```python
from build123d import *
from OCP.BRepFilletAPI import BRepFilletAPI_MakeChamfer

# Parameters (mm, degrees)
SKETCH1_W          = 20.32
SKETCH1_H          = 40.64
EXTRUDE1_DEPTH     = 29.2
SKETCH2_W          = 20.32
SKETCH2_H          = 40.64
EXTRUDE2_DEPTH     = 2.38125
SKETCH3_W          = 20.32
SKETCH3_H          = 40.64
EXTRUDE3_DEPTH     = 8.2
EXTRUDE6_DEPTH     = 0.635
CHAMFER2_SIZE      = 2.54
CHAMFER2_SIZE2     = 1.466469684
FILLET1_R          = 1.016
FILLET2_R          = 1.524
SKETCH9_W          = 6.35
SKETCH9_H          = 2.54
EXTRUDE8_DEPTH     = 2.38125
SKETCH10_W         = 5.08
SKETCH10_H         = 1.27
CUT_EXTRUDE1_DEPTH = 2.38125
SKETCH_1_R         = 6.5
EXTRUDE_1_DEPTH    = 2
EXTRUDE_1_TAPER    = 9
FILLET_1_R         = 0.5
SKETCH_2_R         = 2.5
EXTRUDE_2_DEPTH    = 4


with BuildPart() as part:
    # Sketch1 → Extrude1 (new body)
    with BuildSketch(Plane(origin=(0, 0, 0), x_dir=(1, 0, 0), z_dir=(0, 1, 0))):
        with Locations((0, -10.16)):
            Rectangle(SKETCH1_W, SKETCH1_H)
    extrude(amount=EXTRUDE1_DEPTH)

    # Sketch2 → Extrude2 (add)
    with BuildSketch(Plane(origin=(0, 29.2, 0), x_dir=(-1, 0, 0), z_dir=(0, 1, 0))):
        with Locations((0, 10.16)):
            Rectangle(SKETCH2_W, SKETCH2_H)
        with BuildLine():
            ThreePointArc((6.731, -15.51418631), (5.08, -11.7094), (3.429, -15.51418631))
            Line((3.429, -15.51418631), (3.429, -16.4846))
            Line((3.429, -16.4846), (-3.429, -16.4846))
            Line((-3.429, -16.4846), (-3.429, -15.51418631))
            ThreePointArc((-3.429, -15.51418631), (-5.08, -11.7094), (-6.731, -15.51418631))
            Line((-6.731, -15.51418631), (-6.731, -16.4846))
            Line((-6.731, -16.4846), (-10.16, -16.4846))
            Line((-10.16, -16.4846), (-10.16, -10.16))
            Line((-10.16, -10.16), (10.16, -10.16))
            Line((10.16, -10.16), (10.16, -16.4846))
            Line((10.16, -16.4846), (6.731, -16.4846))
            Line((6.731, -16.4846), (6.731, -15.51418631))
        make_face()
        with BuildLine():
            ThreePointArc((-6.731, 35.83418631), (-5.08, 32.0294), (-3.429, 35.83418631))
            Line((-3.429, 35.83418631), (-3.429, 36.8046))
            Line((-3.429, 36.8046), (3.429, 36.8046))
            Line((3.429, 36.8046), (3.429, 35.83418631))
            ThreePointArc((3.429, 35.83418631), (5.08, 32.0294), (6.731, 35.83418631))
            Line((6.731, 35.83418631), (6.731, 36.8046))
            Line((6.731, 36.8046), (10.16, 36.8046))
            Line((10.16, 36.8046), (10.16, 30.48))
            Line((10.16, 30.48), (-10.16, 30.48))
            Line((-10.16, 30.48), (-10.16, 36.8046))
            Line((-10.16, 36.8046), (-6.731, 36.8046))
            Line((-6.731, 36.8046), (-6.731, 35.83418631))
        make_face()
    extrude(amount=EXTRUDE2_DEPTH)

    # Sketch3 → Extrude3 (add)
    with BuildSketch(Plane(origin=(0, 31.58125, 0), x_dir=(-1, 0, 0), z_dir=(0, 1, 0))):
        with Locations((0, 10.16)):
            Rectangle(SKETCH3_W, SKETCH3_H)
    extrude(amount=EXTRUDE3_DEPTH)

    # Sketch7 → Extrude6 (add, symmetric)
    with BuildSketch(Plane(origin=(0, 0, 0), x_dir=(0, 0, -1), z_dir=(1, 0, 0))):
        Polygon((15.494, 31.58125), (12.954, 33.35925), (10.16, 33.35925), (10.16, 31.58125), align=None)
    extrude6 = extrude(amount=EXTRUDE6_DEPTH, both=True)

    # Mirror1: Extrude6 across plane
    add(extrude6.mirror(Plane(origin=(0, 0, 10.16), x_dir=(1, 0, 0), z_dir=(0, 0, -1))))

    # Chamfer2: one chamfer whose edges measure the first distance from different faces: ONE call of the kernel's chamfer builder (chamfer() names one face for all edges)
    chamfer2_edges_1 = [part.edges().sort_by_distance(p)[0] for p in [
        (0, 0, -10.16),
    ]]
    chamfer2_side_1 = [part.faces().sort_by_distance(p)[0] for p in [
        (0, 14.6, -10.16),
    ]]
    chamfer2_edges_2 = [part.edges().sort_by_distance(p)[0] for p in [
        (0, 0, 30.48),
    ]]
    chamfer2_side_2 = [part.faces().sort_by_distance(p)[0] for p in [
        (0, 14.6, 30.48),
    ]]
    chamfer2 = BRepFilletAPI_MakeChamfer(part.part.solid().wrapped)
    for e in chamfer2_edges_1:
        chamfer2.Add(CHAMFER2_SIZE, CHAMFER2_SIZE2, e.wrapped, chamfer2_side_1[0].wrapped)  # the first distance lies on this face
    for e in chamfer2_edges_2:
        chamfer2.Add(CHAMFER2_SIZE, CHAMFER2_SIZE2, e.wrapped, chamfer2_side_2[0].wrapped)  # the first distance lies on this face
    add(Compound.cast(chamfer2.Shape()), mode=Mode.REPLACE)

    # Fillet1
    fillet1_edges = [part.edges().sort_by_distance(p)[0] for p in [
        (-10.16, 35.68125, -10.16),
        (10.16, 35.68125, -10.16),
        (10.16, 35.68125, 30.48),
        (10.16, 0, 10.16),
        (10.16, 1.27, -9.426765158),
        (10.16, 15.87, -10.16),
        (0, 0, -8.693530316),
        (0, 2.54, -10.16),
        (-10.16, 15.87, -10.16),
        (-10.16, 1.27, -9.426765158),
        (10.16, 15.87, 30.48),
        (10.16, 1.27, 29.746765158),
        (0, 2.54, 30.48),
        (-10.16, 0, 10.16),
        (0, 0, 29.013530316),
        (-10.16, 1.27, 29.746765158),
        (-10.16, 15.87, 30.48),
        (-10.16, 35.68125, 30.48),
    ]]
    fillet(fillet1_edges, radius=FILLET1_R)

    # Fillet2
    fillet2_edges = [part.edges().sort_by_distance(p)[0] for p in [
        (-10.16, 30.390625, 36.8046),
        (10.16, 30.390625, 36.8046),
        (-10.16, 30.390625, -16.4846),
        (10.16, 30.390625, -16.4846),
    ]]
    fillet(fillet2_edges, radius=FILLET2_R)

    # Sketch9 → Extrude8 (add)
    with BuildSketch(Plane(origin=(0, 0, -10.16), x_dir=(-1, 0, 0), z_dir=(0, 0, -1))):
        with Locations((0, 11.27)):
            Rectangle(SKETCH9_W, SKETCH9_H)
    extrude(amount=EXTRUDE8_DEPTH)

    # Sketch10 → Cut-Extrude1 (cut)
    with BuildSketch(Plane(origin=(0, 0, -12.54125), x_dir=(-1, 0, 0), z_dir=(0, 0, -1))):
        with Locations((0, 11.27)):
            Rectangle(SKETCH10_W, SKETCH10_H)
    extrude(amount=-CUT_EXTRUDE1_DEPTH, mode=Mode.SUBTRACT)

    # Эскиз1 → Вытянуть1 (add)
    with BuildSketch(Plane(origin=(0, 39.78125, 0), x_dir=(1, 0, 0), z_dir=(0, 1, 0))):
        with Locations((0, 1.16)):
            Circle(SKETCH_1_R)
    extrude(amount=EXTRUDE_1_DEPTH, taper=EXTRUDE_1_TAPER)

    # Скругление1
    fillet_1_edges = [part.edges().sort_by_distance(p)[0] for p in [
        (-6.5, 39.78125, -1.16),
    ]]
    fillet(fillet_1_edges, radius=FILLET_1_R)

    # Эскиз2 → Вытянуть2 (add)
    with BuildSketch(Plane(origin=(0, 41.78125, 0), x_dir=(1, 0, 0), z_dir=(0, 1, 0))):
        with Locations(Location((0, 1.16, 0), (0, 0, 270))):
            Circle(SKETCH_2_R)
    extrude(amount=EXTRUDE_2_DEPTH)


solid = part.part
```
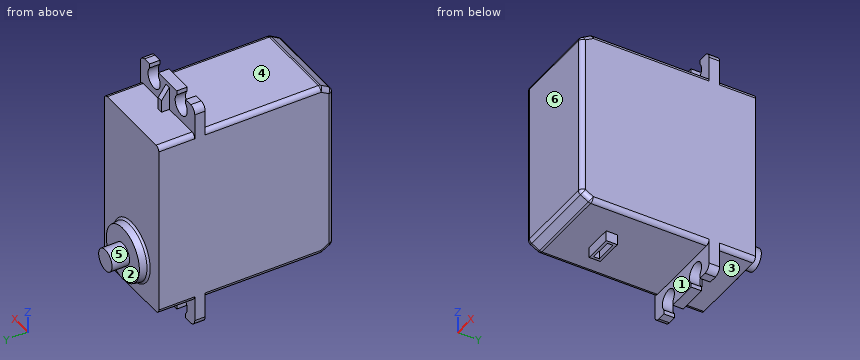
CAD build for the part. Positions are in the model's coordinates, mm. Face numbers are marked on the shaded views. A direction names the side the tool comes from. Round coordinates to 2 decimals unless told otherwise and drop trailing zeros. Write each loop counter-clockwise with the first axis right and the second up, starting at its lowest first coordinate (ties: lowest second). Pieces come first, ordered by that corner, then holes. Notation, with made-up numbers: (28, 60) - (75, 60) arc R24 ccw to (75, 93) - close; hole circle Ø9 at (88, 25). An arc over 180 degrees is marked (long way). Return JSON: item names as keys, results as strings. Group by question number.
Item 1: Band-saw the part on C-C on z = -13.97. List the corners of the cut face in (x, y) (3 decimals).
Item 2: Probe probe 1 along X at (y, z) = (30.9, -13.97); probe 2 along X at (y, z) = (30, -13); probe 3 along Z at (x, y) = (7.25, 32). List the from-to ranges inside material, lowest first.
Item 3: Band-saw the part on A-A on y = 38. List the corners of the cut face in (x, z).
Item 4: Flat gauge pins, fed straight in: pin 1 Ø2.5 at (x, z) = (1, -11.5) entering from -Y; pin 2 Ø10 at (x, y) = (0, 9.5) entering from -Z; pin 3 Ø3 at (x, y) = (0, 27.5) entering from +Z. Where does each tip first touch, or does it go through?
Item 5: Band-saw the part on B-B on z = 24.5. List the corners of the cut face in (x, y).
Item 6: 3-axis set-ups, long thin cutter, end or side, ignore diameter. For the marked faces 4, 5 and 6: which of +Z, -Z, +X, -X, +Y, -Y reach the whole face in a straight line?
Item 7: Mould opens along Y. For the marked faces 1, 2 and 3 say: +Y half, -Y half, draft (parallel to the pull), parting line (faces both ways), or undercut.
Resolved:
{
 "1": {"outline": "(-10.16, 29.2) - (-7.341, 29.2) - (-7.341, 31.581) - (-10.16, 31.581) - close; (-2.819, 29.2) - (2.819, 29.2) - (2.819, 31.581) - (0.635, 31.581) - (0.635, 32.648) - (-0.635, 32.648) - (-0.635, 31.581) - (-2.819, 31.581) - close; (7.341, 29.2) - (10.16, 29.2) - (10.16, 31.581) - (7.341, 31.581) - close"},
 "2": {"probe 1": "x = -10.16 to -7.34, -2.82 to 2.82, 7.34 to 10.16", "probe 2": "x = -10.16 to -7.12, -3.04 to 3.04, 7.12 to 10.16", "probe 3": "z = -10.16 to 30.48"},
 "3": {"outline": "(-10.16, -9.14) arc R1.02 ccw to (-9.14, -10.16) - (9.14, -10.16) arc R1.02 ccw to (10.16, -9.14) - (10.16, 29.46) arc R1.02 ccw to (9.14, 30.48) - (-9.14, 30.48) arc R1.02 ccw to (-10.16, 29.46) - close"},
 "4": {"pin 1": "stops at y = 10", "pin 2": "stops at z = -12.54", "pin 3": "stops at z = 30.48"},
 "5": {"outline": "(-10.16, 1.02) arc R1.02 ccw to (-9.14, 0) - (9.14, 0) arc R1.02 ccw to (10.16, 1.02) - (10.16, 39.78) - (-10.16, 39.78) - close"},
 "6": {"face 4": "+Z, +X, -X, -Y", "face 5": "+Y", "face 6": "+Z, -Z, +X, -X, -Y"},
 "7": {"face 1": "undercut", "face 2": "+Y half", "face 3": "draft"}
}
